Here's how the part is built. I have some questions about the finished solid (model axes, mm). A direction names the side the tool comes from. Round coordinates to 2 decimals unless told otherwise and drop trailing zeros. Order: outer loops, then holes, each group sorted by start corner. A loop starts at its lowest first (then second) coordinate and runs counter-clockwise, first axis right, second up. Notation, with made-up numbers: (-12.5, 24.5) -> (27.5, 24.5) arc R19 ccw to (27.5, 51.5) -> close; hole circle Ø1 at (-32, 5). An arc over 180 degrees is marked (long way). Use a Markdown table: item, result. Add a question column.
(1) Thinking about a two-plate mould opening in X: for faces 3 (the face through (257.336, 493.695, 0.385)), 4 (the face through (43, 433, -27.5)), 5 (the face through (50.272, 456.87, -0.385)), 6 (the face through (152.365, 661.446, -0.385)), which applies, pulls with the +X half, pulls with the -X half, needs draft (parallel to the pull), parting line crosses it, or undercut?
(2) I'm going to push flat-ended pins straight in: P1, Ø1.5, axis at x = 208, z = 18.5, coming from the -Y side; P2, Ø1, axis at x = 230, z = 18.5, coming from the -Y side; P3, Ø4, axis at y = 346, z = 21, coming from the -X side. Where does each tip first touch, or does it pass through?
(3) I want a section at B-B, the plane y = 414. Please give me the cut outline in (x, z), then the cut area to 3 significant figures.
(4) If I drill on probe 1 along X at (y, z) = (516.5, 19); probe 2 along X at (y, z) = (504, 24); probe 3 along Y at (x, z) = (161, -16.5), over which ranges is the centre line in solid material (lowest first)?
(5) I want a section at A-A, the plane x = 182. Please give me the cut outline in (y, z), then the cut area to 3 significant figures.
(6) On a 3-axis mill with a long thin cutter (end or side, diameter ignored), from which of +Z, -Z, +X, -X, +Y, -Y can I reach the whole of each face in a straight line? I mean faces 1 (the face through (199.83, 288.81, 0.38)), 2 (the face through (197.7, 290.98, -0.38)). Say none if no direction works.
Solid Edge part; units mm, degrees
sketch "Sketch1" plane through (0, 0, 0) normal (0, 0, 1) x (1, 0, 0)
  arc A0 (93.177716, 611.594363) -> (215.822462, 613.945088) centre (154.85041, 594.492351) cw
  line L0 (292.066721, 374.967452) -> (215.822462, 613.945088)
  arc A1 (292.066721, 356.730512) -> (292.066721, 374.967452) centre (263.486072, 365.848982) ccw
  line L1 (105.942903, 227.051431) -> (292.066721, 356.730512)
  arc A2 (6.148455, 297.752399) -> (105.942903, 227.051431) centre (68.784785, 280.383169) ccw
  line L2 (93.177716, 611.594363) -> (6.148455, 297.752399)
sketch "Sketch2" plane through (93.177716, 611.594363, 0) normal (-0.2672189, -0.9636358, 0) x (-0.9636358, 0.2672189, 0)
  line L0 (0, -27.5) -> (3, -27.5)
  line L1 (3, -27.5) -> (3, 27.5)
  line L2 (3, 27.5) -> (0, 27.5)
  line L3 (0, 27.5) -> (0, -27.5)
  dimension "D1" = 3
  dimension "D2" = 3
sweep "SweptProtrusion1" add profiles "Sketch2" path "Sketch1"
properties material "Aluminum, 6061-T6"
Taken from the geometry:
| question | item | result |
|---|---|---|
| 1 | face 3 | pulls with the +X half |
| 1 | face 4 | needs draft |
| 1 | face 5 | undercut |
| 1 | face 6 | parting line crosses it |
| 2 | P1 | stops at y = 293.98 |
| 2 | P2 | stops at y = 309.48 |
| 2 | P3 | stops at x = 15.86 |
| 3 | outline | (35.27, -27.5) -> (38.38, -27.5) -> (38.38, 27.5) -> (35.27, 27.5) -> close; (279.61, -27.5) -> (282.76, -27.5) -> (282.76, 27.5) -> (279.61, 27.5) -> close |
| 3 | area | 344 mm2 |
| 4 | probe 1 | x = 63.69 to 66.81, 246.91 to 250.06 |
| 4 | probe 2 | x = 60.23 to 63.34, 250.9 to 254.05 |
| 4 | probe 3 | y = 261.76 to 265.41, 658.2 to 661.21 |
| 5 | outline | (276.39, -27.5) -> (280.04, -27.5) -> (280.04, 27.5) -> (276.39, 27.5) -> close; (652.45, -27.5) -> (655.75, -27.5) -> (655.75, 27.5) -> (652.45, 27.5) -> close |
| 5 | area | 382 mm2 |
| 6 | face 1 | +Z, -Z, +X, -Y |
| 6 | face 2 | +Z, -Z |
